Part print with two shaded views. Sizes in mm from the minimum x, y, z corner. A direction names the side the tool comes from. Give positions to 0.01 mm unless a question says otherwise; leave off trailing zeros. Order: outer loops, then holes, each group sorted by start corner. A loop starts at its lowest first (then second) coordinate and runs counter-clockwise, first axis right, second up. Notation, with made-up numbers: M 21.25,-13 L 33.25,-13 A14 cw 33.25,11 Z; hole C 19,2.25 d5. An arc over 180 degrees is marked long. Answer as CSV lines item,"result".
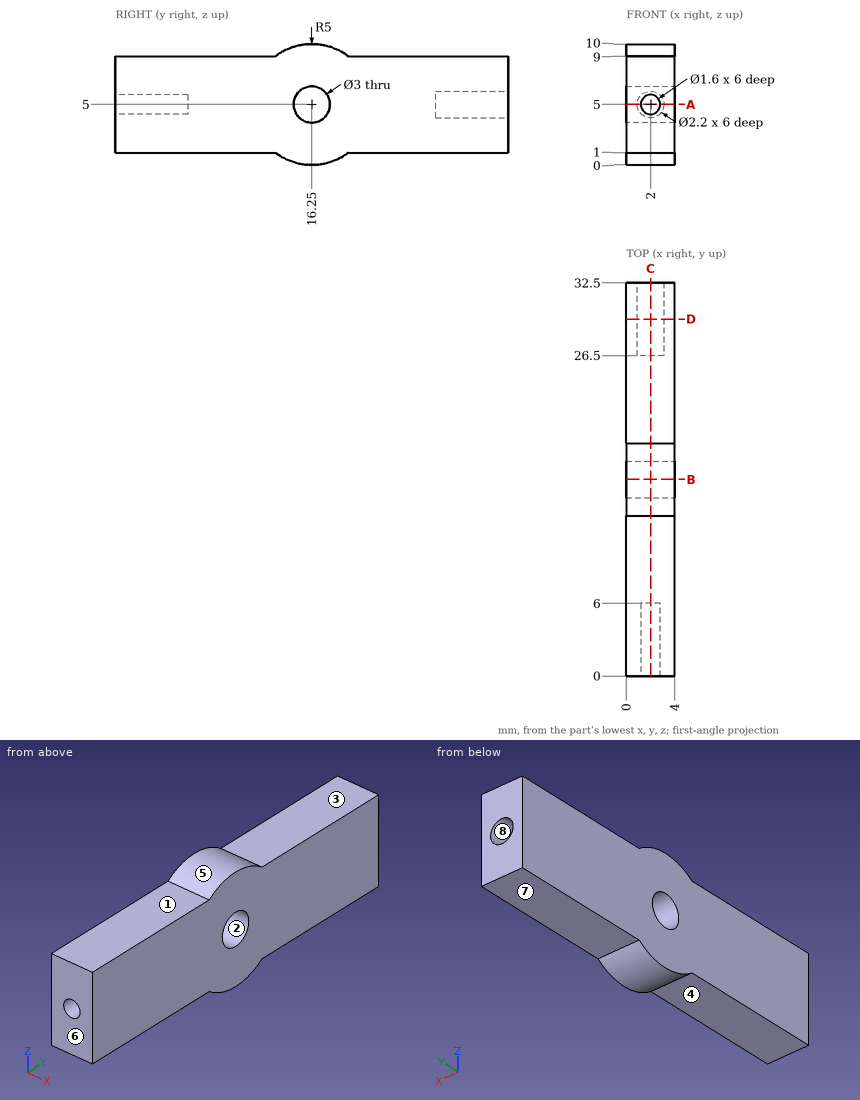
Item 1: Band-saw the part on B-B (y = 16.25). Give the cut face in (x, z), and give its area (3 significant figures).
Geometry says:
outline,"M 0,0 L 4,0 L 4,3.5 L 0,3.5 Z; M 0,6.5 L 4,6.5 L 4,10 L 0,10 Z"
area,"28.0 mm2"
Item 2: Pull direction Z, two halves, no side cores. Call the marked faces 6, 7 and 8: released by +Z, released by -Z, zero draft, split by the parting line, or undercut.
Geometry says:
face 6,"zero draft"
face 7,"released by -Z"
face 8,"undercut"
Item 3: Band-saw the part on D-D (y = 29.5). Give the cut face in (x, z), and give its area (3 significant figures).
Geometry says:
outline,"M 0,1 L 4,1 L 4,9 L 0,9 Z; hole C 2,5 d2.2"
area,"28.2 mm2"
Item 4: 3-axis set-ups, long thin cutter, end or side, ignore diameter. For the marked faces 1, 2, 3, 4 and 5: which of +Z, -Z, +X, -X, +Y, -Y reach the whole face in a straight line?
Geometry says:
face 1,"+Z, +X, -X, -Y"
face 2,"+X, -X"
face 3,"+Z, +X, -X, +Y"
face 4,"-Z, +X, -X, -Y"
face 5,"+Z, +X, -X"
Item 5: Band-saw the part on A-A (z = 5). Give the cut face in (x, y).
Geometry says:
outline,"M 0,0 L 1.2,0 L 1.2,6 L 2.8,6 L 2.8,0 L 4,0 L 4,14.75 L 0,14.75 Z; M 0,17.75 L 4,17.75 L 4,32.5 L 3.1,32.5 L 3.1,26.5 L 0.9,26.5 L 0.9,32.5 L 0,32.5 Z"
Item 6: Probe line 1 along Z through (x, y) = (2, 29.35); line 2 along Y through (x, z) = (2.75, 5); line 3 along Z through (x, y) = (2, 2.75). List the from-to ranges inside material, lowest first. Write a range as from..to.
Geometry says:
line 1,"z = 1..3.9, 6.1..9"
line 2,"y = 6..14.75, 17.75..26.5"
line 3,"z = 1..4.2, 5.8..9"
Item 7: Band-saw the part on C-C (x = 2). Give the cut face in (y, z).
Geometry says:
outline,"M 0,1 L 13.25,1 A5 ccw 19.25,1 L 32.5,1 L 32.5,3.9 L 26.5,3.9 L 26.5,6.1 L 32.5,6.1 L 32.5,9 L 19.25,9 A5 ccw 13.25,9 L 0,9 L 0,5.8 L 6,5.8 L 6,4.2 L 0,4.2 Z; hole C 16.25,5 d3"
Item 8: Drop flat-ended pins along their axis: pin 1 (1.8 mm diameter, centred on x = 1.5, z = 5.5, fed in from +Y); pin 2 (2 mm diameter, centred on x = 1.5, y = 4, fed in from +Z); pin 3 (1.8 mm diameter, centred on x = 2, z = 5, fed in from +Y). Give the stop position or say it passes through.
Geometry says:
pin 1,"stops at y = 32.5"
pin 2,"stops at z = 9"
pin 3,"stops at y = 26.5"
